from build123d import *

# Parameters (mm, degrees)
BOSS_EXTRU_1_DEPTH      = 5
BOSS_EXTRU_2_DEPTH      = 14
ESQUISSE5_R             = 1.8
ENL_V_MAT_EXTRU_1_DEPTH = 56.088510189
BOSS_EXTRU_3_DEPTH      = 15
ESQUISSE7_R             = 1.6
ENL_V_MAT_EXTRU_2_DEPTH = 66.014675864
ESQUISSE3_4_OUTSIDE_W   = 40.383
ESQUISSE3_4_OUTSIDE_H   = 112.114
ENL_V_MAT_EXTRU_5_DEPTH = 58.617219265
NERVURE2_REACH          = 65.559
ESQUISSE9_WALL_W        = 156.631593158
ESQUISSE9_WALL_H        = 24
ENL_V_MAT_EXTRU_6_DEPTH = 2.5


with BuildPart() as part:
    # Esquisse1 → Boss.-Extru.1 (new body)
    with BuildSketch(Plane.XY):
        Polygon((-10.105828541, -19), (-10.105828541, 19), (-17.072507544, 45), (-13.966679003, 45), (-7, 19), (0, 19), (0, -19), (-7, -19), (-13.966679003, -45), (-17.072507544, -45), align=None)
    extrude(amount=BOSS_EXTRU_1_DEPTH)

    # Esquisse2 → Boss.-Extru.2 (add)
    with BuildSketch(Plane.XY.offset(5)):
        Polygon((-17.072507544, 45), (-10.105828541, 19), (-10.105828541, -19), (-17.072507544, -45), (-13.966679003, -45), (-7, -19), (-7, 19), (-13.966679003, 45), align=None)
    extrude(amount=BOSS_EXTRU_2_DEPTH)

    # Esquisse4 → Lissage1 section 0
    with BuildSketch(Plane.XY.offset(19)):
        with BuildLine():
            Line((-13.966679003, -45), (-7, -19))
            Line((-7, -19), (-7, 19))
            Line((-7, 19), (-13.966679003, 45))
            Line((-13.966679003, 45), (-17.072507544, 45))
            Line((-17.072507544, 45), (-10.105828541, 19))
            Line((-10.105828541, 19), (-10.105828541, -19))
            Line((-10.105828541, -19), (-17.072507544, -45))
            Line((-17.072507544, -45), (-13.966679003, -45))
        make_face()
    # Esquisse3 → Lissage1 section 1
    with BuildSketch(Plane.XY.offset(31)):
        with BuildLine():
            Line((-18.268659967, 45), (-15.162831426, 45))
            Line((-15.162831426, 45), (-9, 22))
            Line((-9, 22), (-9, -22))
            Line((-9, -22), (-15.162831426, -45))
            Line((-15.162831426, -45), (-18.268659967, -45))
            Line((-18.268659967, -45), (-12.105828541, -22))
            Line((-12.105828541, -22), (-12.105828541, 22))
            Line((-12.105828541, 22), (-18.268659967, 45))
        make_face()
    loft()

    # Esquisse5 → Enlèv. mat.-Extru.1 (cut, through all)
    with BuildSketch(Plane.XY.offset(5)):
        with Locations(Location((-3.5, -15.5, 0), (0, 0, 180))):
            Circle(ESQUISSE5_R)
        with Locations((-3.5, 15.5)):
            Circle(ESQUISSE5_R)
    extrude(amount=-ENL_V_MAT_EXTRU_1_DEPTH, mode=Mode.SUBTRACT)

    # Esquisse6 → Boss.-Extru.3 (add)
    with BuildSketch(Plane.XY.offset(31)):
        Polygon((-9, 45), (-18.268659967, 45), (-12.105828541, 22), (-12.105828541, -22), (-18.268659967, -45), (-9, -45), align=None)
    extrude(amount=BOSS_EXTRU_3_DEPTH)

    # Esquisse7 → Enlèv. mat.-Extru.2 (cut, through all)
    with BuildSketch(Plane.ZY.offset(9)):
        with BuildLine():
            ThreePointArc((40.764205464, 19.762918321), (38.632351614, 15.188236146), (34.145898034, 17.5))
            Line((34.145898034, 17.5), (33.145898034, 17.5))
            Line((33.145898034, 17.5), (31, 15))
            Line((31, 15), (31, -15))
            Line((31, -15), (33.145898034, -17.5))
            Line((33.145898034, -17.5), (34.145898034, -17.5))
            ThreePointArc((34.145898034, -17.5), (38.632351614, -15.188236146), (40.764205464, -19.762918321))
            Line((40.764205464, -19.762918321), (31, -45))
            Line((31, -45), (46, -45))
            Line((46, -45), (46, 45))
            Line((46, 45), (31, 45))
            Line((31, 45), (40.764205464, 19.762918321))
        make_face()
        with Locations(Location((37.5, 18.5, 0), (0, 0, 180))):
            Circle(ESQUISSE7_R)
        with Locations(Location((37.5, -18.5, 0), (0, 0, 90))):
            Circle(ESQUISSE7_R)
    extrude(amount=ENL_V_MAT_EXTRU_2_DEPTH, mode=Mode.SUBTRACT)

    # Esquisse3<4> outside → Enlèv. mat.-Extru.5 (cut, through all)
    with BuildSketch(Plane.XY.offset(31)):
        with Locations((-9.1345, 0)):
            Rectangle(ESQUISSE3_4_OUTSIDE_W, ESQUISSE3_4_OUTSIDE_H)
        Polygon((-18.268659967, 45), (-15.162831426, 45), (-9, 22), (-9, -22), (-15.162831426, -45), (-18.268659967, -45), (-12.105828541, -22), (-12.105828541, 22), align=None, mode=Mode.SUBTRACT)
    extrude(amount=ENL_V_MAT_EXTRU_5_DEPTH, mode=Mode.SUBTRACT)

    # Esquisse9 wall → Nervure2 (add, up to next)
    with BuildSketch(Plane(origin=(-4.5, 0, 18), x_dir=(-0.327110563883, 0, 0.94498607344), z_dir=(-0.94498607344, 0, -0.327110563883)), mode=Mode.PRIVATE) as nervure2_sk1:
        Rectangle(ESQUISSE9_WALL_W, ESQUISSE9_WALL_H)
    nervure2_tool1 = extrude(nervure2_sk1.sketch, amount=NERVURE2_REACH, mode=Mode.PRIVATE) - part.part
    add(nervure2_tool1.solids().sort_by_distance((-4.5, 0, 18))[0])

    # Esquisse10 → Enlèv. mat.-Extru.6 (cut)
    with BuildSketch(Plane.XY.offset(5)):
        Polygon((-5.079865302, 18.225165248), (-1.939526432, 18.225165248), (-0.369356996, 15.50555201), (-1.920134698, 12.774834752), (-5.060473568, 12.774834752), (-6.630643004, 15.49444799), align=None)
        Polygon((-6.630643004, -15.49444799), (-5.079865302, -18.225165248), (-1.939526432, -18.225165248), (-0.369356996, -15.50555201), (-1.920134698, -12.774834752), (-5.060473568, -12.774834752), align=None)
    extrude(amount=-ENL_V_MAT_EXTRU_6_DEPTH, mode=Mode.SUBTRACT)


solid = part.part
Input: part model. Units: mm. Frame: model coordinates. A direction names the side the tool comes from. Give positions to 0.01 mm unless a question says otherwise; leave off trailing zeros. Write each loop counter-clockwise with the first axis right and the second up, starting at its lowest first coordinate (ties: lowest second). Pieces come first, ordered by that corner, then holes.
Q1. Set-up query: faces 4 (the face through (-1, 17, 5)), 5 (the face through (-11, 0, 31)), 6 (the face through (-12.106, -19, 35)), 7 (the face through (-5.835, -14.116, 3.768)), 8 (the face through (-11.354, -30.783, 34.398)). Return all of +Z, -Z, +X, -X, +Y, -Y with unobstructed straight access to the full face (end or side cutting, diameter ignored); none if empty.
Q2. Material intervals for probe 1 along Y at (x, z) = (-3.5, 1.65); probe 2 along Y at (x, z) = (-4.25, 3.5); probe 3 along X at (y, z) = (-15.5, 1.8), sorted ascending.
Q3. Pull-direction query (Y, two-part tool) for faces 1 (the face through (0, 0, 2)), 2 (the face through (-4, 19, 2)), 3 (the face through (-3, -12.775, 4)); classes: pulls with the +Y half, pulls with the -Y half, needs draft (parallel to the pull), parting line crosses it, or undercut.
Q4. First-contact query: P1, Ø5.5, axis at y = 14.5, z = 10.5, coming from the +X side; P2, Ø12, axis at y = -3.5, z = 28, coming from the -X side; P3, Ø8, axis at y = -30, z = 12.5, coming from the -X side. Flat tips, straight axial feed; report the tip coordinate or a pass-through.
Q5. Section A-A, the plane z = 37.5. Output: boundary loops of the cut face in (x, y).
Q6. Section B-B, the plane x = -3.5. Output: boundary loops of the cut face in (y, z), plus the area to 3 significant figures.
Filled in:
1. face 4: +Z, +X, +Y
1. face 5: +Z, +X, -X
1. face 6: +Z, -Z, -X
1. face 7: +Z
1. face 8: +Z, +X, -Y
2. probe 1: y = -19 to -17.3, -13.7 to 13.7, 17.3 to 19
2. probe 2: y = -19 to -18.23, -12.77 to 12.77, 18.23 to 19
2. probe 3: x = -10.11 to -5.3, -1.7 to 0
3. face 1: needs draft
3. face 2: pulls with the +Y half
3. face 3: undercut
4. P1: stops at x = -1.51
4. P2: stops at x = -12.11
4. P3: stops at x = -14.13
5. outline: (-13.77, -28.2) - (-10.66, -28.2) - (-9, -22) - (-9, -20.1) - (-12.11, -20.1) - (-12.11, -22) - close; (-13.77, 28.2) - (-12.11, 22) - (-12.11, 20.1) - (-9, 20.1) - (-9, 22) - (-10.66, 28.2) - close; (-12.11, -16.9) - (-9, -16.9) - (-9, -15) - (-12.11, -15) - close; (-12.11, 15) - (-9, 15) - (-9, 16.9) - (-12.11, 16.9) - close
6. outline: (-19, 0) - (-17.3, 0) - (-17.3, 2.5) - (-18.23, 2.5) - (-18.23, 5) - (-19, 5) - close; (-13.7, 0) - (13.7, 0) - (13.7, 2.5) - (12.77, 2.5) - (12.77, 5) - (12, 5) - (12, 15.11) - (-12, 15.11) - (-12, 5) - (-12.77, 5) - (-12.77, 2.5) - (-13.7, 2.5) - close; (17.3, 0) - (19, 0) - (19, 5) - (18.23, 5) - (18.23, 2.5) - (17.3, 2.5) - close
6. area: 387 mm2
